from build123d import *

# Parameters (mm, degrees)
BOSS_EXTRUDE1_DEPTH = 3
CUT_EXTRUDE1_DEPTH  = 3
FILLET1_R           = 10
SKETCH3_R           = 9
CUT_EXTRUDE2_DEPTH  = 3


with BuildPart() as part:
    # Sketch1 → Boss-Extrude1 (new body)
    with BuildSketch(Plane(origin=(0, 0, 0), x_dir=(0, 0, -1), z_dir=(1, 0, 0))):
        Polygon((0, 0), (11.910798094, 6.158004928), (42.739414765, 12.383521095), (90.106781804, 14.033136775), (135.887385092, 10.713704644), (219.287488067, -1.876713431), (270.057015241, -12.532639482), (283.823146281, -14.792882614), (299.988096251, -15.517362165), (299.988096251, -40), (0, -40), align=None)
    extrude(amount=BOSS_EXTRUDE1_DEPTH)

    # Sketch2 → Cut-Extrude1 (cut)
    with BuildSketch(Plane(origin=(3, 0, 0), x_dir=(0, 0, -1), z_dir=(1, 0, 0))):
        with BuildLine():
            Line((35, -40), (35, -38))
            ThreePointArc((35, -38), (37.928932188, -30.928932188), (45, -28))
            Line((45, -28), (225, -28))
            ThreePointArc((225, -28), (232.071067812, -30.928932188), (235, -38))
            Line((235, -38), (235, -40))
            Line((235, -40), (35, -40))
        make_face()
    extrude(amount=-CUT_EXTRUDE1_DEPTH, mode=Mode.SUBTRACT)

    # Fillet1
    fillet1_edges = [part.edges().sort_by_distance(p)[0] for p in [
        (1.5, -40, -235),
        (1.5, -40, -35),
    ]]
    fillet(fillet1_edges, radius=FILLET1_R)

    # Sketch3 → Cut-Extrude2 (cut)
    with BuildSketch(Plane(origin=(3, 0, 0), x_dir=(0, 0, -1), z_dir=(1, 0, 0))):
        with Locations((73.81, -3.27)):
            Circle(SKETCH3_R)
    extrude(amount=-CUT_EXTRUDE2_DEPTH, mode=Mode.SUBTRACT)


solid = part.part
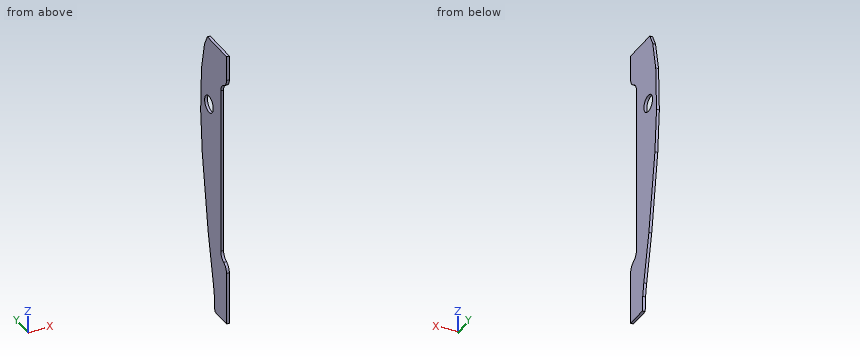
Geometry check sheet. Reference: the model listing, model coordinates, mm. Give positions to 0.01 mm unless a question says otherwise; leave off trailing zeros. Order: outer loops, then holes, each group sorted by start corner. A loop starts at its lowest first (then second) coordinate and runs counter-clockwise, first axis right, second up.
1. Sectioned sample at A-A (z = -73.81). Record the boundary of the cut face in (x, y), then the cut area to 3 significant figures.
Completed:
outline: (0, -28) - (3, -28) - (3, -12.27) - (0, -12.27) - close; (0, 5.73) - (3, 5.73) - (3, 13.47) - (0, 13.47) - close
area: 70.4 mm2
2. Sectioned sample at B-B (z = -210). Record the boundary of the cut face in (x, y).
Completed:
outline: (0, -28) - (3, -28) - (3, -0.47) - (0, -0.47) - close
3. Scan lines: line 1 (Z direction, x = 0.85, y = -32.5); line 2 (Y direction, x = 0.75, z = -73.81); line 3 (Y direction, x = 1.6, z = -209). Record each from-to range of solid material in increasing order.
Completed:
line 1: z = -299.99 to -233.35, -36.65 to 0
line 2: y = -28 to -12.27, 5.73 to 13.47
line 3: y = -28 to -0.32
4. Depth check by flat-ended pin: pin 1 (1.5 mm diameter, centred on x = 1.5, z = -160, fed in from -Y). Enter the tip coordinate at first touch or a pass-through.
Completed:
pin 1: stops at y = -28
